For this review, take the finished solid that the model builds, in its own axes (mm). Round coordinates to 2 decimals unless told otherwise and drop trailing zeros. Write each loop counter-clockwise with the first axis right and the second up, starting at its lowest first coordinate (ties: lowest second). Pieces come first, ordered by that corner, then holes. Notation, with made-up numbers: (0.25, -35) -> (10.25, -35) arc R9 cw to (10.25, -30) -> close; hole circle Ø8 at (63, 70.25). An arc over 180 degrees is marked (long way). Answer in a Markdown table with one row per item. Add a question column.
Autodesk Inventor part; units mm, degrees
ref_plane "YZ Plane" through (0, 0, 0) normal (1, 0, 0) x (0, 1, 0)
ref_plane "XZ Plane" through (0, 0, 0) normal (0, 1, 0) x (-1, 0, 0)
ref_plane "XY Plane" through (0, 0, 0) normal (0, 0, 1) x (1, 0, 0)
sketch "Sketch1" plane through (0, 0, 0) normal (0, 0, 1) x (1, 0, 0)
  line L0 (0, 0) -> (203.2, 0)
  line L1 (203.2, 0) -> (203.2, 7.62)
  line L2 (203.2, 7.62) -> (0, 7.62)
  line L3 (0, 7.62) -> (0, 0)
  dimension "d0" = 7.62
  dimension "d1" = 203.2
revolve "Revolution1" add sketch "Sketch1" angle 180 about axis through (0, 7.62, 0) along (0, 1, 0)
chamfer "Chamfer1" distance 2.54 angle 45 1 edges at (-101.6, 7.62, 0)
properties part number "shelf-backplate"
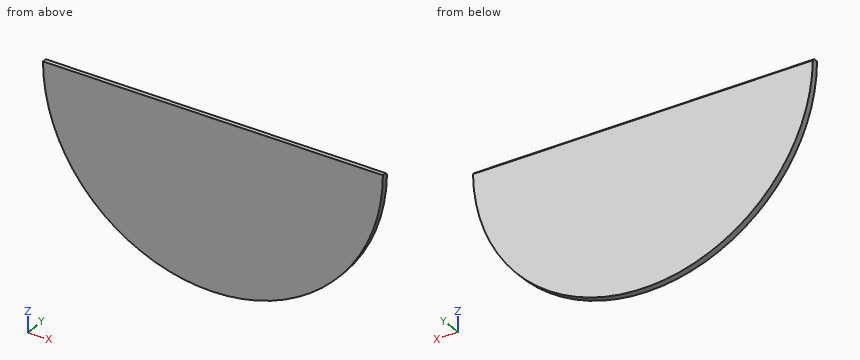
1. Clearance check with a flat-ended pin moving along its axis: pin 1 Ø1 at (y, z) = (6.5, -41.5) entering from +X. State where the tip first meets the part, or that it passes through.
2. We need section A-A (y = 3.75). Write out the cut boundary in (x, z).
3. For L1, parallel to Z at x = -78.5, y = 5; L2, parallel to X at y = 4, z = -141.5; L3, parallel to X at y = 1.25, z = -19, list the stretches that pass through material, from the lowest coordinate up. Write a range as [from, to].
4. We need section B-B (x = -130). Write out the cut boundary in (y, z).
5. We need section D-D (x = 109.5). Write out the cut boundary in (y, z), plus the area to 3 significant figures.
6. We need section C-C (z = -44.5). Write out the cut boundary in (x, y).
Response:
| question | item | result |
|---|---|---|
| 1 | pin 1 | x = 199.02 |
| 2 | outline | (-203.2, 0) arc R203.2 ccw to (203.2, 0) -> close |
| 3 | L1 | [-187.42, 0] |
| 3 | L2 | [-145.84, 145.84] |
| 3 | L3 | [-202.31, 202.31] |
| 4 | outline | (0, -156.17) -> (7.62, -156.17) -> (7.62, -2.54) -> (5.08, 0) -> (0, 0) -> close |
| 5 | outline | (0, -171.17) -> (7.62, -171.17) -> (7.62, -2.54) -> (5.08, 0) -> (0, 0) -> close |
| 5 | area | 1,300 mm2 |
| 6 | outline | (-198.27, 0) -> (198.27, 0) -> (198.27, 7.62) -> (-198.27, 7.62) -> close |
